Part model, mm, in its own coordinate system. A direction names the side the tool comes from. Coordinates: 2 decimals unless noted, no trailing zeros. Write each loop counter-clockwise with the first axis right and the second up, starting at its lowest first coordinate (ties: lowest second). Pieces come first, ordered by that corner, then holes. Notation, with made-up numbers: M 52.25,43.25 L 70.25,43.25 A20 cw 70.25,60.25 Z; hole C 4,-2.75 d3. An arc over 180 degrees is marked long. Use a Markdown table: item, result. Add a question column.
Q1. Pin check, flat tips, straight feed: pin 1 Ø15.5 at (x, y) = (125, 125) entering from +Z; pin 2 Ø11 at (x, y) = (112.5, 112.5) entering from -Z; pin 3 Ø6 at (y, z) = (20.5, -24) entering from +X; pin 4 Ø3.5 at (x, y) = (-124, 126) entering from +Z. Stop position of each tip, or through.
Q2. Mould opens along X. For faces 4 (the conical face through (137.027, 136.656, -26.181)), 5 (the cylindrical face through (-116.92, 116.56, -24.93)), 6 (the conical face through (-137.027, -136.656, -26.181)) say: released by +X, released by -X, zero draft, split by the parting line, or undercut.
Q3. Wall check: L1, parallel to Y at x = 125, z = -4; L2, parallel to Y at x = 112.5, z = -22.75; L3, parallel to Z at x = -134.5, y = -134. Give the ranges that are in metal, low to high. Write a range as from..to.
Q4. Slice it at A-A on x = 112.5. Write the cut outline in (y, z).
Q5. Tool access for faces 1 (the flat face through (112, 113, -20)), 2 (the flat face through (125, -125, -10)), 3 (the conical face through (136.656, -137.027, -26.181)): list every direction of +Z, -Z, +X, -X, +Y, -Y with a clear straight run to the whole face (end or side of a thin tool).
from build123d import *

# Parameters (mm, degrees)
F0_R     = 6
F1_DEPTH = 30
F2_SIZE2 = 10
F2_SIZE  = 10
F3_DEPTH = 10
F4_DEPTH = 20


with BuildPart() as f1:
    # F0 (on Top) → F1 (new body)
    with BuildSketch(Plane.XY):
        with BuildLine():
            ThreePointArc((150, 120), (141.213203, 141.213203), (120, 150))
            Line((120, 150), (-120, 150))
            ThreePointArc((-120, 150), (-141.213203, 141.213203), (-150, 120))
            Line((-150, 120), (-150, -120))
            ThreePointArc((-150, -120), (-141.213203, -141.213203), (-120, -150))
            Line((-120, -150), (120, -150))
            ThreePointArc((120, -150), (141.213203, -141.213203), (150, -120))
            Line((150, -120), (150, 120))
        make_face()
        with Locations((-125, -125)):
            Circle(F0_R, mode=Mode.SUBTRACT)
        with Locations((-112.5, -112.5)):
            Circle(F0_R, mode=Mode.SUBTRACT)
        with Locations((125, -125)):
            Circle(F0_R, mode=Mode.SUBTRACT)
        with Locations((112.5, -112.5)):
            Circle(F0_R, mode=Mode.SUBTRACT)
        with Locations((-125, 125)):
            Circle(F0_R, mode=Mode.SUBTRACT)
        with Locations((-112.5, 112.5)):
            Circle(F0_R, mode=Mode.SUBTRACT)
        with Locations((112.5, 112.5)):
            Circle(F0_R, mode=Mode.SUBTRACT)
        with Locations((125, 125)):
            Circle(F0_R, mode=Mode.SUBTRACT)
        with Locations((-125, 125)):
            Circle(F0_R)
        with Locations((125, 125)):
            Circle(F0_R)
        with Locations((125, -125)):
            Circle(F0_R)
        with Locations((-125, -125)):
            Circle(F0_R)
    extrude(amount=-F1_DEPTH)

    # F2
    f2_edges = [f1.edges().sort_by_distance(p)[0] for p in [
        (0, 150, -30),
    ]]
    chamfer(f2_edges, length=F2_SIZE, length2=F2_SIZE2)

    # F0 (on Top) → F3 (cut)
    with BuildSketch(Plane.XY):
        with Locations((-125, 125)):
            Circle(F0_R)
        with Locations((125, 125)):
            Circle(F0_R)
        with Locations((-125, -125)):
            Circle(F0_R)
        with Locations((125, -125)):
            Circle(F0_R)
    extrude(amount=-F3_DEPTH, mode=Mode.SUBTRACT)

    # F0 (on Top) → F4 (join)
    with BuildSketch(Plane.XY):
        with Locations((-112.5, 112.5)):
            Circle(F0_R)
        with Locations((112.5, 112.5)):
            Circle(F0_R)
        with Locations((112.5, -112.5)):
            Circle(F0_R)
        with Locations((-112.5, -112.5)):
            Circle(F0_R)
    extrude(amount=-F4_DEPTH)


solid = f1.part
Recorded:
| question | item | result |
|---|---|---|
| 1 | pin 1 | z = 0 |
| 1 | pin 2 | z = -20 |
| 1 | pin 3 | x = 149 |
| 1 | pin 4 | z = -10 |
| 2 | face 4 | released by +X |
| 2 | face 5 | undercut |
| 2 | face 6 | released by -X |
| 3 | L1 | -149.58..-131, -119..119, 131..149.58 |
| 3 | L2 | -147.25..-118.5, -106.5..106.5, 118.5..147.25 |
| 3 | L3 | -29.84..0 |
| 4 | outline | M -150,-20 L -140,-30 L -118.5,-30 L -118.5,-20 L -106.5,-20 L -106.5,-30 L 106.5,-30 L 106.5,-20 L 118.5,-20 L 118.5,-30 L 140,-30 L 150,-20 L 150,0 L -150,0 Z |
| 5 | face 1 | -Z |
| 5 | face 2 | +Z |
| 5 | face 3 | -Z, +X, -Y |
